Geometry: final body of the model. Coordinates: model frame, mm. Face numbers are marked on the shaded views. A direction names the side the tool comes from. Round coordinates to 2 decimals unless told otherwise and drop trailing zeros. Loops run counter-clockwise (first coordinate to the right, second up) from the corner with the lowest first, then second, coordinate; pieces in that order, holes last. Notation, with made-up numbers: (10, 27) - (18, 27) arc R17 ccw to (18, 54) - close; hole circle Ø10 at (-16, 73.25). An arc over 180 degrees is marked (long way). Answer in a Markdown table with one row per item. Add a question column.
from build123d import *

# Parameters (mm, degrees)
SKETCH1_R           = 247.65
SKETCH1_R_2         = 187.325
BOSS_EXTRUDE1_DEPTH = 63.5
BOSS_EXTRUDE2_START = 12.7
SKETCH2_R           = 247.65
BOSS_EXTRUDE2_DEPTH = 12.7
BOSS_EXTRUDE3_START = 82.55
BOSS_EXTRUDE3_DEPTH = 69.85
CUT_EXTRUDE1_REACH  = 447.403
SKETCH4_R           = 12.7


with BuildPart() as part:
    # Sketch1 → Boss-Extrude1 (new body)
    with BuildSketch(Plane(origin=(0, 0, 0), x_dir=(1, 0, 0), z_dir=(0, 1, 0))):
        with Locations(Location((0, 0, 0), (0, 0, 270))):
            Circle(SKETCH1_R)
        with Locations(Location((0, 0, 0), (0, 0, 270))):
            Circle(SKETCH1_R_2, mode=Mode.SUBTRACT)
    extrude(amount=BOSS_EXTRUDE1_DEPTH)

    # Sketch2 → Boss-Extrude2 (add)
    # profile 1 of 6: a face of its own
    with BuildSketch(Plane.XZ.offset(BOSS_EXTRUDE2_START)):
        with Locations(Location((0, 0, 0), (0, 0, 270))):
            Circle(SKETCH2_R)
        with BuildLine():
            Line((-206.375, -113.236721076), (-206.375, 113.236721076))
            Line((-206.375, 113.236721076), (-149.225, 113.236721076))
            ThreePointArc((-149.225, 113.236721076), (0, 187.325), (149.225, 113.236721076))
            Line((149.225, 113.236721076), (206.375, 113.236721076))
            Line((206.375, 113.236721076), (206.375, -113.236721076))
            Line((206.375, -113.236721076), (149.225, -113.236721076))
            ThreePointArc((149.225, -113.236721076), (0, -187.325), (-149.225, -113.236721076))
            Line((-149.225, -113.236721076), (-206.375, -113.236721076))
        make_face(mode=Mode.SUBTRACT)
    # profile 2 of 6: a face of its own
    with BuildSketch(Plane.XZ.offset(BOSS_EXTRUDE2_START)):
        with BuildLine():
            Line((206.375, 113.236721076), (149.225, 113.236721076))
            ThreePointArc((149.225, 113.236721076), (177.544682756, 59.737268518), (187.325, 0))
            ThreePointArc((187.325, 0), (177.544682756, -59.737268518), (149.225, -113.236721076))
            Line((149.225, -113.236721076), (206.375, -113.236721076))
            Line((206.375, -113.236721076), (206.375, 113.236721076))
        make_face()
    # profile 3 of 6: a face of its own
    with BuildSketch(Plane.XZ.offset(BOSS_EXTRUDE2_START)):
        with BuildLine():
            ThreePointArc((187.325, 0), (177.544682756, 59.737268518), (149.225, 113.236721076))
            Line((149.225, 113.236721076), (149.225, -113.236721076))
            ThreePointArc((149.225, -113.236721076), (177.544682756, -59.737268518), (187.325, 0))
        make_face()
    # profile 4 of 6: a face of its own
    with BuildSketch(Plane.XZ.offset(BOSS_EXTRUDE2_START)):
        with BuildLine():
            Line((-149.225, -113.236721076), (-149.225, 113.236721076))
            ThreePointArc((-149.225, 113.236721076), (-187.325, 0), (-149.225, -113.236721076))
        make_face()
    # profile 5 of 6: a face of its own
    with BuildSketch(Plane.XZ.offset(BOSS_EXTRUDE2_START)):
        with BuildLine():
            ThreePointArc((149.225, 113.236721076), (0, 187.325), (-149.225, 113.236721076))
            Line((-149.225, 113.236721076), (-149.225, -113.236721076))
            ThreePointArc((-149.225, -113.236721076), (0, -187.325), (149.225, -113.236721076))
            Line((149.225, -113.236721076), (149.225, 113.236721076))
        make_face()
    # profile 6 of 6: a face of its own
    with BuildSketch(Plane.XZ.offset(BOSS_EXTRUDE2_START)):
        with BuildLine():
            Line((-149.225, 113.236721076), (-206.375, 113.236721076))
            Line((-206.375, 113.236721076), (-206.375, -113.236721076))
            Line((-206.375, -113.236721076), (-149.225, -113.236721076))
            ThreePointArc((-149.225, -113.236721076), (-187.325, 0), (-149.225, 113.236721076))
        make_face()
    extrude(amount=-BOSS_EXTRUDE2_DEPTH)

    # Sketch2<3> → Boss-Extrude3 (add)
    with BuildSketch(Plane.XZ.offset(BOSS_EXTRUDE3_START)):
        with BuildLine():
            Line((-149.225, -113.236721076), (-149.225, 113.236721076))
            ThreePointArc((-149.225, 113.236721076), (-187.325, 0), (-149.225, -113.236721076))
        make_face()
        with BuildLine():
            Line((-149.225, 113.236721076), (-206.375, 113.236721076))
            Line((-206.375, 113.236721076), (-206.375, -113.236721076))
            Line((-206.375, -113.236721076), (-149.225, -113.236721076))
            ThreePointArc((-149.225, -113.236721076), (-187.325, 0), (-149.225, 113.236721076))
        make_face()
        with BuildLine():
            Line((206.375, 113.236721076), (149.225, 113.236721076))
            ThreePointArc((149.225, 113.236721076), (177.544682756, 59.737268518), (187.325, 0))
            ThreePointArc((187.325, 0), (177.544682756, -59.737268518), (149.225, -113.236721076))
            Line((149.225, -113.236721076), (206.375, -113.236721076))
            Line((206.375, -113.236721076), (206.375, 113.236721076))
        make_face()
        with BuildLine():
            ThreePointArc((187.325, 0), (177.544682756, 59.737268518), (149.225, 113.236721076))
            Line((149.225, 113.236721076), (149.225, -113.236721076))
            ThreePointArc((149.225, -113.236721076), (177.544682756, -59.737268518), (187.325, 0))
        make_face()
    extrude(amount=-BOSS_EXTRUDE3_DEPTH)

    # Sketch4 → Cut-Extrude1 (cut, up to next)
    with BuildSketch(Plane.XY.offset(113.236721076), mode=Mode.PRIVATE) as cut_extrude1_sk1:
        with Locations((177.8, -50.8)):
            Circle(SKETCH4_R)
    cut_extrude1_tool1 = extrude(cut_extrude1_sk1.sketch, amount=-CUT_EXTRUDE1_REACH, mode=Mode.PRIVATE) & part.part
    # Sketch4 → Cut-Extrude1 (cut, up to next)
    with BuildSketch(Plane.XY.offset(113.236721076), mode=Mode.PRIVATE) as cut_extrude1_sk2:
        with Locations((-177.8, -50.8)):
            Circle(SKETCH4_R)
    cut_extrude1_tool2 = extrude(cut_extrude1_sk2.sketch, amount=-CUT_EXTRUDE1_REACH, mode=Mode.PRIVATE) & part.part
    add(cut_extrude1_tool1.solids().sort_by_distance((177.8, -50.8, 113.236721))[0], mode=Mode.SUBTRACT)
    add(cut_extrude1_tool2.solids().sort_by_distance((-177.8, -50.8, 113.236721))[0], mode=Mode.SUBTRACT)


solid = part.part
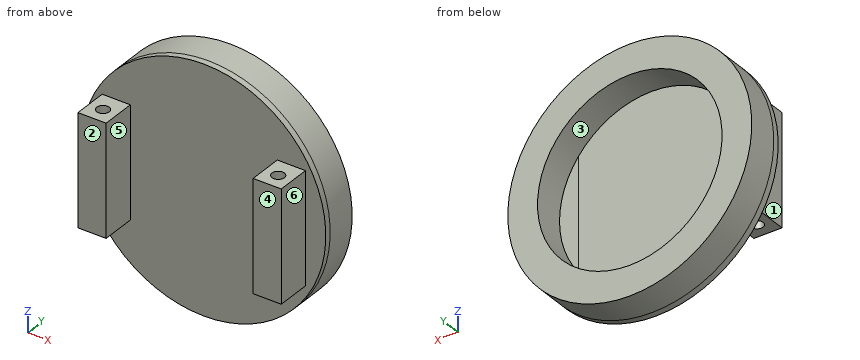
1) Contact query for flat-ended pins moving along their axis: pin 1 Ø21 at (y, z) = (-45.5, -49) entering from +X (3 decimals); pin 2 Ø10 at (x, y) = (61, 29) entering from +Z; pin 3 Ø4 at (x, z) = (95.5, 63) entering from +Y. Output: stop coordinate, or through.
2) Section B-B, the plane x = 0. Return the cut outline in (y, z) (3 decimals).
3) Pull-direction query (X, two-part tool) for the marked faces 4, 5 and 6; classes: pulls with the +X half, pulls with the -X half, needs draft (parallel to the pull), parting line crosses it, or undercut.
4) Material intervals for line 1 along X through (y, z) = (-50, 61) (3 decimals); line 2 along X through (y, z) = (-49, -21.5) (3 decimals); line 3 along X through (y, z) = (29, 0) (3 decimals), sorted ascending. Write a range as from..to.
5) Reachability of the marked faces 1, 2 and 3 from +Z, -Z, +X, -X, +Y, -Y: full face, straight path, thin tool, end or side. Return the list, or none.
6) Section D-D, the plane y = 43. Return the cut outline in (x, z) (3 decimals), and give its area (3 significant figures).
7) Section A-A, the plane x = -173. Return the cut outline in (y, z), and give its area (3 significant figures).
8) Section C-C, the plane z = 19. Return the cut outline in (x, y) (3 decimals), and give its area (3 significant figures).
Evaluation:
| question | item | result |
|---|---|---|
| 1 | pin 1 | stops at x = 206.375 |
| 1 | pin 2 | stops at z = 241.24 |
| 1 | pin 3 | stops at y = 0 |
| 2 | outline | (-12.7, -247.65) - (63.5, -247.65) - (63.5, -187.325) - (0, -187.325) - (0, 187.325) - (63.5, 187.325) - (63.5, 247.65) - (-12.7, 247.65) - close |
| 3 | face 4 | needs draft |
| 3 | face 5 | undercut |
| 3 | face 6 | pulls with the +X half |
| 4 | line 1 | x = -206.375..-190.475, -165.125..-149.225, 149.225..165.125, 190.475..206.375 |
| 4 | line 2 | x = -206.375..-190.372, -165.228..-149.225, 149.225..165.228, 190.372..206.375 |
| 4 | line 3 | x = -247.65..-187.325, 187.325..247.65 |
| 5 | face 1 | +Z, -Z, -X, -Y |
| 5 | face 2 | +Z, -Z, +X, -X, -Y |
| 5 | face 3 | +Y |
| 6 | outline | circle Ø495.3 at (0, 0); hole circle Ø374.65 at (0, 0) |
| 6 | area | 82,400 mm² |
| 7 | outline | (-82.55, -113.24) - (-62.56, -113.24) - (-62.56, 113.24) - (-82.55, 113.24) - close; (-39.04, -113.24) - (-12.7, -113.24) - (-12.7, -177.2) - (63.5, -177.2) - (63.5, -71.84) - (0, -71.84) - (0, 71.84) - (63.5, 71.84) - (63.5, 177.2) - (-12.7, 177.2) - (-12.7, 113.24) - (-39.04, 113.24) - close |
| 7 | area | 28,400 mm² |
| 8 | outline | (-246.92, -12.7) - (-206.375, -12.7) - (-206.375, -82.55) - (-149.225, -82.55) - (-149.225, -12.7) - (149.225, -12.7) - (149.225, -82.55) - (206.375, -82.55) - (206.375, -12.7) - (246.92, -12.7) - (246.92, 63.5) - (186.359, 63.5) - (186.359, 0) - (-186.359, 0) - (-186.359, 63.5) - (-246.92, 63.5) - close; hole circle Ø25.4 at (-177.8, -50.8); hole circle Ø25.4 at (177.8, -50.8) |
| 8 | area | 20,900 mm² |
